```python
from build123d import *

# Parameters (mm, degrees)
SKETCH1_W           = 70
SKETCH1_H           = 38
SKETCH1_R           = 1
BOSS_EXTRUDE1_DEPTH = 10
SKETCH2_R           = 1.25
CUT_EXTRUDE1_DEPTH  = 12


with BuildPart() as part:
    # Sketch1 → Boss-Extrude1 (new body)
    with BuildSketch(Plane.XY):
        with Locations((-4.613461538, -5.005769231)):
            Rectangle(SKETCH1_W, SKETCH1_H)
        with Locations((-21.613461538, 11.994230769)):
            Circle(SKETCH1_R, mode=Mode.SUBTRACT)
        with Locations((12.386538462, 11.994230769)):
            Circle(SKETCH1_R, mode=Mode.SUBTRACT)
        with Locations((12.386538462, -22.005769231)):
            Circle(SKETCH1_R, mode=Mode.SUBTRACT)
        with Locations((-21.613461538, -22.005769231)):
            Circle(SKETCH1_R, mode=Mode.SUBTRACT)
    extrude(amount=BOSS_EXTRUDE1_DEPTH)

    # Sketch2 → Cut-Extrude1 (cut)
    with BuildSketch(Plane(origin=(30.386538462, 0, 0), x_dir=(0, 0, -1), z_dir=(1, 0, 0))):
        with Locations((-5, 9.994230769)):
            Circle(SKETCH2_R)
        with Locations((-5, -20.005769231)):
            Circle(SKETCH2_R)
    cut_extrude1 = extrude(amount=-CUT_EXTRUDE1_DEPTH, mode=Mode.SUBTRACT)

    # Mirror1: Cut-Extrude1 across plane
    add(cut_extrude1.mirror(Plane.ZY.offset(4.613461538)), mode=Mode.SUBTRACT)


solid = part.part
```
Source: CAD feature listing. Evaluate the final solid. Frame: model axes, mm. A direction names the side the tool comes from. Coordinates: 2 decimals unless noted, no trailing zeros. Order: outer loops, then holes, each group sorted by start corner. A loop starts at its lowest first (then second) coordinate and runs counter-clockwise, first axis right, second up. Notation, with made-up numbers: (27.5, -25) - (78.5, -25) arc R16 cw to (78.5, -12) - close; hole circle Ø9 at (8.5, -23). An arc over 180 degrees is marked (long way). One line per item, written item: value.
1) Ray query, line 1 (Y direction, x = 22.25, z = 5); line 2 (X direction, y = 12, z = 7.25); line 3 (Y direction, x = 26, z = 5.75). Return the intervals inside material, ascending. Write a range as [from, to].
Computed values:
line 1: y = [-24.01, -21.26], [-18.76, 8.74], [11.24, 13.99]
line 2: x = [-39.61, -22.61], [-20.61, 11.39], [13.39, 30.39]
line 3: y = [-24.01, -21.01], [-19.01, 8.99], [10.99, 13.99]
2) Contact query for flat-ended pins moving along their axis: pin 1 (2 mm diameter, centred on y = 9.99, z = 5, fed in from +X); pin 2 (3 mm diameter, centred on y = -20.01, z = 5, fed in from -X). Output: stop coordinate, or through.
Computed values:
pin 1: stops at x = 18.39
pin 2: stops at x = -39.61
3) Cut plane A-A on z = 5. Output: boundary loops of the cut face in (x, y).
Computed values:
outline: (-39.61, -24.01) - (30.39, -24.01) - (30.39, -21.26) - (18.39, -21.26) - (18.39, -18.76) - (30.39, -18.76) - (30.39, 8.74) - (18.39, 8.74) - (18.39, 11.24) - (30.39, 11.24) - (30.39, 13.99) - (-39.61, 13.99) - (-39.61, 11.24) - (-27.61, 11.24) - (-27.61, 8.74) - (-39.61, 8.74) - (-39.61, -18.76) - (-27.61, -18.76) - (-27.61, -21.26) - (-39.61, -21.26) - close; hole circle Ø2 at (-21.61, -22.01); hole circle Ø2 at (-21.61, 11.99); hole circle Ø2 at (12.39, -22.01); hole circle Ø2 at (12.39, 11.99)
4) Mould query, pull axis Y, two halves, no side actions, for faces 1 (the face through (-39.613, -5, 5)), 2 (the face through (-5, -24.006, 5)), 3 (the face through (24.47, 10.05, 6.25)). Classes: released by +Y, released by -Y, zero draft, split by the parting line, or undercut.
Computed values:
face 1: zero draft
face 2: released by -Y
face 3: undercut
5) Reachability of faces 4 (the face through (-27.613, 10, 5)), 5 (the face through (18.387, -20, 5)), 6 (the face through (30.387, -5, 5)) from +Z, -Z, +X, -X, +Y, -Y: full face, straight path, thin tool, end or side. Return the list, or none.
Computed values:
face 4: -X
face 5: +X
face 6: +Z, -Z, +X, +Y, -Y
